```python
from build123d import *

# Parameters (mm, degrees)
SKETCH012_W             = 1.6
SKETCH012_H             = 8.3
EXTRUDE011_DEPTH        = 1.6
SKETCH008_R             = 4
EXTRUDE007_DEPTH        = 4
BODY004_PLACEMENT_ANGLE = 180


with BuildPart() as extrude011:
    # Sketch012 → Extrude011 (new body)
    with BuildSketch(Plane.XY.offset(5)):
        with Locations((14, 4.15)):
            Rectangle(SKETCH012_W, SKETCH012_H)
        with Locations((18, 4.15)):
            Rectangle(SKETCH012_W, SKETCH012_H)
        with Locations((-10, 4.15)):
            Rectangle(SKETCH012_W, SKETCH012_H)
        with Locations((-14, 4.15)):
            Rectangle(SKETCH012_W, SKETCH012_H)
    extrude(amount=-EXTRUDE011_DEPTH)


with BuildPart() as extrude011_1:
    # Extrude011 placement: moved
    add(extrude011.part.moved(Location((0, 0, -1))))


with BuildPart() as cut:
    # Sketch008 → Extrude007 (new body)
    with BuildSketch(Plane.XY):
        with BuildLine():
            ThreePointArc((3.3, 0), (0, 3.3), (-3.3, 0))
            Line((-3.3, 0), (-19, 0))
            Line((-19, 0), (-19, 19))
            Line((-19, 19), (19, 19))
            Line((19, 19), (19, 0))
            Line((3.3, 0), (19, 0))
        make_face()
        with Locations((-13, 13)):
            Circle(SKETCH008_R, mode=Mode.SUBTRACT)
        with Locations((13, 13)):
            Circle(SKETCH008_R, mode=Mode.SUBTRACT)
    extrude(amount=EXTRUDE007_DEPTH)

    # Cut: cut Extrude011
    add(extrude011_1.part, mode=Mode.SUBTRACT)


with BuildPart() as revolve001:
    # Sketch014 → Revolve001 (revolve)
    with BuildSketch(Plane.XZ):
        Polygon((-11, 0), (-11, -10), (-10, -10), (-10, -3), (-7, 0), align=None)
    revolve(axis=Axis((0, 0, 0), (0, 0, 1)))


with BuildPart() as body:
    # Body base: copy of Cut
    add(cut.part)


with BuildPart() as body004:
    # Part__Mirroring: instance of Body
    add(body.part.mirror(Plane(origin=(0, 0, 0), x_dir=(1, 0, 0), z_dir=(0, 1, 0))))

    # Fusion004: union Cut, Revolve001
    add(cut.part)
    add(revolve001.part)


with BuildPart() as body004_1:
    # Body004 placement: moved
    add(body004.part.moved(Location((0, 0, -42))).rotate(Axis((0, 0, -42), (0, 1, 0)), BODY004_PLACEMENT_ANGLE))


solid = body004_1.part
```
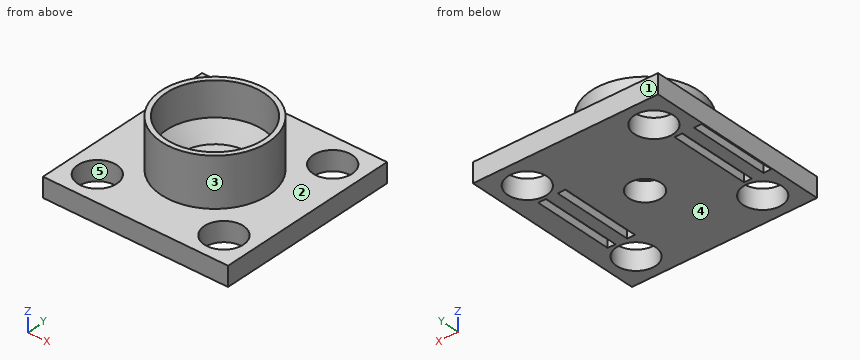
Source: CAD feature listing. Evaluate the final solid. Frame: model axes, mm. Face numbers are marked on the shaded views. A direction names the side the tool comes from. Give positions to 0.01 mm unless a question says otherwise; leave off trailing zeros. Order: outer loops, then holes, each group sorted by start corner. A loop starts at its lowest first (then second) coordinate and runs counter-clockwise, first axis right, second up. Notation, with made-up numbers: (5.5, 27.25) -> (52.5, 27.25) arc R31 cw to (52.5, 66.25) -> close; hole circle Ø1 at (51.25, 41). An arc over 180 degrees is marked (long way). Use a Markdown table: item, result.
Q1. Material intervals for line 1 (X direction, y = -13, z = -44.6); line 2 (X direction, y = -10.5, z = -45), sorted ascending. Write a range as [from, to].
A:
| item | result |
|---|---|
| line 1 | [-19, -17], [-9, 9], [17, 19] |
| line 2 | [-19, -16.12], [-9.88, 9.88], [16.12, 19] |
Q2. Section C-C (y = 13). Return the cut outline in (x, z), and give its area (3 significant figures).
A:
| item | result |
|---|---|
| outline | (-19, -46) -> (-17, -46) -> (-17, -42) -> (-19, -42) -> close; (-9, -46) -> (9, -46) -> (9, -42) -> (-9, -42) -> close; (17, -46) -> (19, -46) -> (19, -42) -> (17, -42) -> close |
| area | 88.0 mm^2 |
Q3. First-contact query: P1, Ø11, axis at x = 1.5, y = -2, coming from the +Z side; P2, Ø1.5, axis at x = 3.5, z = -37.5, coming from the +Y side; P3, Ø2, axis at x = -1.5, z = -37, coming from the -Y side. Flat tips, straight axial feed; report the tip coordinate or a pass-through.
A:
| item | result |
|---|---|
| P1 | z = -41 |
| P2 | y = 10.65 |
| P3 | y = -10.99 |
Q4. Access query for the marked faces 1 and 2. Directions: +Z, -Z, +X, -X, +Y, -Y. A direction counts if a zero-diameter tool reaches every point of the face in a straight line with its end or side. Return the directions, or none.
A:
| item | result |
|---|---|
| face 1 | +Z, -Z, +X, -X, +Y |
| face 2 | +Z |
Q5. Pull-direction query (Y, two-part tool) for the marked faces 3, 4 and 5; classes: +Y half, -Y half, draft (parallel to the pull), parting line (faces both ways), or undercut.
A:
| item | result |
|---|---|
| face 3 | parting line |
| face 4 | draft |
| face 5 | undercut |
Q6. Section B-B (x = -16). Return the cut outline in (y, z).
A:
| item | result |
|---|---|
| outline | (-19, -46) -> (-15.65, -46) -> (-15.65, -42) -> (-19, -42) -> close; (-10.35, -46) -> (10.35, -46) -> (10.35, -42) -> (-10.35, -42) -> close; (15.65, -46) -> (19, -46) -> (19, -42) -> (15.65, -42) -> close |
Q7. Section D-D (x = 0). Return the cut outline in (y, z).
A:
| item | result |
|---|---|
| outline | (-19, -46) -> (-3.3, -46) -> (-3.3, -42) -> (-7, -42) -> (-10, -39) -> (-10, -32) -> (-11, -32) -> (-11, -42) -> (-19, -42) -> close; (3.3, -46) -> (19, -46) -> (19, -42) -> (11, -42) -> (11, -32) -> (10, -32) -> (10, -39) -> (7, -42) -> (3.3, -42) -> close |
